Autodesk Inventor part; units mm, degrees
ref_plane "YZ Plane" through (0, 0, 0) normal (1, 0, 0) x (0, 1, 0)
ref_plane "XZ Plane" through (0, 0, 0) normal (0, 1, 0) x (-1, 0, 0)
ref_plane "XY Plane" through (0, 0, 0) normal (0, 0, 1) x (1, 0, 0)
sketch "Sketch1" plane through (0, 0, 0) normal (0, 0, 1) x (1, 0, 0)
  point P0 (0, 0)
sketch "Sketch2" plane through (0, 0, 0) normal (0, 0, 1) x (1, 0, 0)
  line L0 (-30, 35) -> (-310, 35)
  line L1 (-310, 35) -> (-310, -35)
  line L2 (-310, -35) -> (-30, -35)
  line L3 (-30, -35) -> (-30, 35)
  line L4 (-310, 35) -> (-30, -35) construction
  line L5 (-30, 35) -> (-310, -35) construction
  line L6 (0, 0) -> (-620.4685, 0)
  point P0 (-170, 0)
  dimension "d0" = 280
  dimension "d1" = 70
  dimension "d2" = 30
extrude "Extrusion1" add sketch "Sketch2" along normal blind 3.65
sketch "Sketch3" plane through (0, 0, 3.65) normal (0, 0, 1) x (1, 0, 0)
  line L0 (-30, 35) -> (-30, -35)
  line L1 (-310, -35) -> (-310, 35)
  line L2 (-30, 0) -> (-310, 0) construction
  line L3 (-42.4613, 25) -> (-37.4613, 25)
  line L4 (-37.4613, 25) -> (-37.4613, -25)
  line L5 (-37.4613, -25) -> (-42.4613, -25)
  line L6 (-42.4613, -25) -> (-42.4613, 25)
  line L7 (-37.4613, 25) -> (-42.4613, -25) construction
  line L8 (-42.4613, 25) -> (-37.4613, -25) construction
  point P0 (0, 0)
  point P1 (-39.9613, 0)
  dimension "d5" = 5
  dimension "d6" = 50
extrude "Extrusion2" add sketch "Sketch3" along normal blind 35.4
sketch "Sketch4" plane through (-42.4613, -25, 3.65) normal (-1, 0, 0) x (0, 0, 1)
  line L0 (35.4, 0) -> (35.4, 50)
  line L1 (0, 50) -> (35.4, 50)
  line L2 (0, 0) -> (0, 50)
  line L3 (0, 0) -> (35.4, 0)
  circle A0 centre (10, 25) radius 10 construction
  line L4 (35.4, 25) -> (-31.6063, 25)
  line L5 (0, 44.8702) -> (15.9582, 33.0312)
  line L6 (0, 5.1298) -> (15.9582, 16.9688)
  circle A1 centre (10, 25) radius 6.4008
  arc A2 (15.9582, 16.9688) -> (15.9582, 33.0312) centre (10, 25) ccw
  line L7 (0, 60) -> (0, -10)
  line L8 (0, 50) -> (35.4, 0) construction
  line L9 (35.4, 50) -> (0, 0) construction
  line L10 (0, -10) -> (0, 60)
  point P0 (-3.65, 25)
  point P1 (17.7, 25)
  point P2 (17.7, 25)
  dimension "d9" = 20
extrude "Extrusion3" cut sketch "Sketch4" against normal through all contours L3 L2 L6 A2 L4 L0 | L4 A2 L5 L2 L1 L0 | A1 L4 | L4 A1
pattern_linear "Rectangular Pattern1" count 2 spacing 265 along (-1, 0, 0) of "Extrusion3", "Extrusion2"
sketch "Sketch5" plane through (0, 0, 3.65) normal (0, 0, 1) x (1, 0, 0)
  line L0 (-30, -35) -> (-310, -35)
  line L1 (-115.953, 3.5653) -> (-116.904, 3.5653)
  line L2 (-116.904, 3.5653) -> (-116.904, -30.6059)
  line L3 (-116.904, -30.6059) -> (-115.953, -30.6059)
  line L4 (-115.953, -30.6059) -> (-115.953, 3.5653)
  line L5 (-85.953, 3.5653) -> (-86.904, 3.5653)
  line L6 (-86.904, 3.5653) -> (-86.904, -30.6059)
  line L7 (-86.904, -30.6059) -> (-85.953, -30.6059)
  line L8 (-85.953, -30.6059) -> (-85.953, 3.5653)
  line L9 (-55.953, 3.5653) -> (-56.904, 3.5653)
  line L10 (-56.904, 3.5653) -> (-56.904, -30.6059)
  line L11 (-56.904, -30.6059) -> (-55.953, -30.6059)
  line L12 (-55.953, -30.6059) -> (-55.953, 3.5653)
  line L13 (-25.953, 3.5653) -> (-26.904, 3.5653)
  line L14 (-26.904, 3.5653) -> (-26.904, -30.6059)
  line L15 (-26.904, -30.6059) -> (-25.953, -30.6059)
  line L16 (-25.953, -30.6059) -> (-25.953, 3.5653)
  line L17 (4.047, 3.5653) -> (3.096, 3.5653)
  line L18 (3.096, 3.5653) -> (3.096, -30.6059)
  line L19 (3.096, -30.6059) -> (4.047, -30.6059)
  line L20 (4.047, -30.6059) -> (4.047, 3.5653)
  line L21 (34.047, 3.5653) -> (33.096, 3.5653)
  line L22 (33.096, 3.5653) -> (33.096, -30.6059)
  line L23 (33.096, -30.6059) -> (34.047, -30.6059)
  line L24 (34.047, -30.6059) -> (34.047, 3.5653)
  point P0 (0, 0)
  dimension "d17" = 30
extrude "Extrusion4" cut sketch "Sketch5" against normal blind 0.25 contours L4 L3 L2 L1
pattern_linear "Rectangular Pattern2" count 6 spacing 30 along (-1, 0, 0) of "Extrusion4"
sketch "Sketch6" plane through (-30, -35, 0) normal (1, 0, 0) x (0, 0, -1)
  line L0 (-3.65, 70) -> (-3.65, 0)
  line L1 (0, 0) -> (-3.65, 0)
  line L2 (0, 0) -> (0, 70)
  line L3 (0, 70) -> (-3.65, 70)
  point P0 (0, 35)
extrude "Extrusion5" add sketch "Sketch6" along normal blind 17.7125
sketch "Sketch7" plane through (0, 0, 3.65) normal (0, 0, 1) x (1, 0, 0)
  line L0 (-266.904, -30.6059) -> (-266.904, 3.5653)
  line L1 (-266.904, 3.5653) -> (-265.953, 3.5653)
  line L2 (-265.953, 3.5653) -> (-265.953, -30.6059)
  line L3 (-265.953, -30.6059) -> (-266.904, -30.6059)
  line L4 (-236.904, -30.6059) -> (-236.904, 3.5653)
  line L5 (-236.904, 3.5653) -> (-235.953, 3.5653)
  line L6 (-235.953, 3.5653) -> (-235.953, -30.6059)
  line L7 (-235.953, -30.6059) -> (-236.904, -30.6059)
  line L8 (-206.904, -30.6059) -> (-206.904, 3.5653)
  line L9 (-206.904, 3.5653) -> (-205.953, 3.5653)
  line L10 (-205.953, 3.5653) -> (-205.953, -30.6059)
  line L11 (-205.953, -30.6059) -> (-206.904, -30.6059)
  line L12 (-176.904, -30.6059) -> (-176.904, 3.5653)
  line L13 (-176.904, 3.5653) -> (-175.953, 3.5653)
  line L14 (-175.953, 3.5653) -> (-175.953, -30.6059)
  line L15 (-175.953, -30.6059) -> (-176.904, -30.6059)
  line L16 (-146.904, -30.6059) -> (-146.904, 3.5653)
  line L17 (-146.904, 3.5653) -> (-145.953, 3.5653)
  line L18 (-145.953, 3.5653) -> (-145.953, -30.6059)
  line L19 (-145.953, -30.6059) -> (-146.904, -30.6059)
  line L20 (-116.904, -30.6059) -> (-116.904, 3.5653)
  line L21 (-116.904, 3.5653) -> (-115.953, 3.5653)
  line L22 (-115.953, 3.5653) -> (-115.953, -30.6059)
  line L23 (-115.953, -30.6059) -> (-116.904, -30.6059)
  line L24 (-302.4613, 19.8702) -> (-302.4613, -19.8702)
  line L25 (-307.4613, -19.8702) -> (-302.4613, -19.8702)
  line L26 (-307.4613, -19.8702) -> (-307.4613, 19.8702)
  line L27 (-307.4613, 19.8702) -> (-302.4613, 19.8702)
  line L28 (-310, 35) -> (-12.2875, 35)
  line L29 (-310, -35) -> (-310, 35)
  line L30 (-12.2875, -35) -> (-310, -35)
  line L31 (-12.2875, -35) -> (-12.2875, 35)
  line L32 (-42.4613, -19.8702) -> (-42.4613, 19.8702)
  line L33 (-42.4613, 19.8702) -> (-37.4613, 19.8702)
  line L34 (-37.4613, 19.8702) -> (-37.4613, -19.8702)
  line L35 (-42.4613, -19.8702) -> (-37.4613, -19.8702)
  line L36 (-12.2875, 35) -> (-12.2875, -35)
  circle A0 centre (-23.1854, 0) radius 10.8979 construction
  line L37 (-12.2875, -35) -> (-12.2875, 35)
  line L38 (-34.0833, 15.009) -> (-19.8116, 10.3625)
  line L39 (-34.0833, 15.009) -> (-34.0833, 35)
  line L40 (-12.2875, 35) -> (-12.2875, 0)
  arc A1 (-12.2875, 0) -> (-19.8116, 10.3625) centre (-23.1854, 0) ccw
  line L41 (-310, 0) -> (-198.3644, 0)
  circle A2 centre (-23.1854, 0) radius 10.8979 construction
  line L42 (-34.0833, -15.009) -> (-19.8116, -10.3625)
  line L43 (-34.0833, -15.009) -> (-34.0833, -35)
  arc A3 (-19.8116, -10.3625) -> (-12.2875, 0) centre (-23.1854, 0) ccw
  line L44 (-34.0833, 15.009) -> (-34.0833, 35)
  line L45 (-12.2875, 35) -> (-12.2875, 0)
  line L46 (-12.2875, -35) -> (-34.0833, -35)
  circle A4 centre (-23.1854, 0) radius 6.826
extrude "Extrusion6" cut sketch "Sketch7" against normal through all contours L28 L31 A1 L38 L39 | L31 L30 L43 L42 A3 | A4
fillet "Fillet1" radius 2 4 edges at (-39.9613, -19.8702, 3.65) (-39.9613, 19.8702, 3.65) (-304.9613, -19.8702, 3.65) (-304.9613, 19.8702, 3.65)
properties part number "ForceMeterCasing"
Source: CAD feature listing. Evaluate the final solid. Frame: model axes, mm. A direction names the side the tool comes from. Coordinates: 2 decimals unless noted, no trailing zeros. Order: outer loops, then holes, each group sorted by start corner. A loop starts at its lowest first (then second) coordinate and runs counter-clockwise, first axis right, second up. Notation, with made-up numbers: (83.5, 36.5) - (87.5, 36.5) arc R29 ccw to (87.5, 56.5) - close; hole circle Ø9 at (66, 59.5). An arc over 180 degrees is marked (long way). One line per item, written item: value.
1) Cut plane C-C on y = 30.5. Output: boundary loops of the cut face in (x, z).
Computed values:
outline: (-310, 0) - (-34.08, 0) - (-34.08, 3.65) - (-310, 3.65) - close
2) Reachability of faces 1 (the face through (-307.461, 0, 7)), 2 (the face through (-39.996, 0.281, 7.255)), 3 (the face through (-302.461, 0, 7)), 4 (the face through (-37.461, 0, 7)) from +Z, -Z, +X, -X, +Y, -Y: full face, straight path, thin tool, end or side. Return the list, or none.
Computed values:
face 1: +Z, -X, +Y, -Y
face 2: +X, -X
face 3: +Z, +Y, -Y
face 4: +Z, +X, +Y, -Y
3) Ray query, line 1 (Z direction, x = -39.25, y = 0); line 2 (X direction, y = -6.5, z = 15.5); line 3 (Y direction, x = -305.9, z = 13.65). Return the intervals inside material, ascending. Write a range as [from, to].
Computed values:
line 1: z = [0, 7.25], [20.05, 23.65]
line 2: x = [-307.46, -302.46], [-42.46, -37.46]
line 3: y = [-12.45, -6.4], [6.4, 12.45]
4) Mould query, pull axis Y, two halves, no side actions, for faces 5 (the face through (-305, -0.13, 23.65)), 6 (the face through (-16.675, 2.05, 1.851)), 7 (the face through (-14.311, 6.325, 1.851)). Classes: released by +Y, released by -Y, zero draft, split by the parting line, or undercut.
Computed values:
face 5: split by the parting line
face 6: undercut
face 7: released by +Y
5) Cut plane B-B on x = -70. Output: boundary loops of the cut face in (y, z).
Computed values:
outline: (-35, 0) - (35, 0) - (35, 3.65) - (-35, 3.65) - close
6) Contact query for flat-ended pins moving along their axis: pin 1 (15.5 mm diameter, centred on x = -23.19, y = 0, fed in from +Z); pin 2 (6 mm diameter, centred on y = -15.5, z = 14.5, fed in from -X); pin 3 (10 mm diameter, centred on y = 24, z = 8.5, fed in from +X). Output: stop coordinate, or through.
Computed values:
pin 1: stops at z = 3.65
pin 2: stops at x = -307.46
pin 3: stops at x = -34.08
7) Cut plane A-A on z = 13.65. Output: boundary loops of the cut face in (x, y).
Computed values:
outline: (-307.46, -12.45) - (-302.46, -12.45) - (-302.46, -6.4) - (-307.46, -6.4) - close; (-307.46, 6.4) - (-302.46, 6.4) - (-302.46, 12.45) - (-307.46, 12.45) - close; (-42.46, -12.45) - (-37.46, -12.45) - (-37.46, -6.4) - (-42.46, -6.4) - close; (-42.46, 6.4) - (-37.46, 6.4) - (-37.46, 12.45) - (-42.46, 12.45) - close
